```python
from build123d import *
from build123d.topology import SkipClean

# Parameters (mm, degrees)
CROQUIS2_R            = 2
CORTAR_EXTRUIR1_DEPTH = 5
REVOLUCI_N2_ANGLE     = 1.5
REVOLUCI_N3_ANGLE     = 1.5
MATRIZC1_COUNT        = 3


with BuildPart() as part:
    # Croquis1 → Revoluci_n1 (revolve)
    with BuildSketch(Plane.XY, mode=Mode.PRIVATE) as revoluci_n1_sk:
        Polygon((0, 56), (0, 90), (3.000002354, 90), (3.000002354, 60.169848481), (10.200002354, 60.169848481), (13.157056275, 57.212794561), (18.657056275, 57.212794561), (41.284473273, 34.585377563), (41.284473273, 32.888321288), (18.16, 56.012794561), (12.66, 56.012794561), (9.70294608, 58.969848481), (3.469848481, 58.969848481), (0.5, 56), align=None)
    revolve(revoluci_n1_sk.sketch.rotate(Axis((-46.033893017, 0, 0), (1, 0, 0)), 90), axis=Axis((-46.033893017, 0, 0), (1, 0, 0)))

    # Croquis2 → Cortar-Extruir1 (cut)
    with SkipClean():  # the faces are left unmerged after this step: merging them gives an invalid solid
        with BuildSketch(Plane.ZY):
            with Locations((63.219854476, 36.5)):
                Circle(CROQUIS2_R)
            with Locations((0, -73)):
                Circle(CROQUIS2_R)
            with Locations((-63.219854476, 36.5)):
                Circle(CROQUIS2_R)
            with BuildLine():
                Line((-14.422814665, 52.006989551), (-15.759006546, 56.825141817))
                ThreePointArc((-15.759006546, 56.825141817), (0, 58.969848481), (15.759006546, 56.825141817))
                Line((15.759006546, 56.825141817), (14.422814665, 52.006989551))
                ThreePointArc((14.422814665, 52.006989551), (0, 53.969848481), (-14.422814665, 52.006989551))
            make_face()
            with BuildLine():
                Line((52.250781458, -13.512970881), (57.09151966, -14.764870902))
                ThreePointArc((57.09151966, -14.764870902), (51.069386842, -29.48492424), (41.332513115, -42.060270916))
                Line((41.332513115, -42.060270916), (37.827966793, -38.49401867))
                ThreePointArc((37.827966793, -38.49401867), (46.739259823, -26.98492424), (52.250781458, -13.512970881))
            make_face()
            with BuildLine():
                Line((-37.827966793, -38.49401867), (-41.332513115, -42.060270916))
                ThreePointArc((-41.332513115, -42.060270916), (-51.069386842, -29.48492424), (-57.09151966, -14.764870902))
                Line((-57.09151966, -14.764870902), (-52.250781458, -13.512970881))
                ThreePointArc((-52.250781458, -13.512970881), (-46.739259823, -26.98492424), (-37.827966793, -38.49401867))
            make_face()
        extrude(amount=-CORTAR_EXTRUIR1_DEPTH, mode=Mode.SUBTRACT)

    # Croquis3 → Revoluci_n2 (revolve)
    with SkipClean():  # the faces are left unmerged after this step: merging them gives an invalid solid
        with BuildSketch(Plane(origin=(0, 0, 0), x_dir=(1, 0, 0), z_dir=(0, -0.9681476403781081, 0.2503800040544404))):
            Polygon((0.5, -56), (12.66, -56.012794561), (9.70294608, -58.969848481), (3.469848481, -58.969848481), align=None)
        revoluci_n2 = revolve(axis=Axis((9.70294608, 0, 0), (1, 0, 0)), revolution_arc=REVOLUCI_N2_ANGLE)

    # Croquis5 → Revoluci_n3 (revolve)
    with SkipClean():  # the faces are left unmerged after this step: merging them gives an invalid solid
        with BuildSketch(Plane(origin=(0, 0, 0), x_dir=(-1, 0, 0), z_dir=(0, -0.9504873560590977, -0.31076323137042167))):
            Polygon((-0.5, 56.012794561), (-3.469848481, 58.969848481), (-9.70294608, 58.969848481), (-12.66, 56.012794561), align=None)
        revoluci_n3 = revolve(axis=Axis((9.70294608, 0, 0), (1, 0, 0)), revolution_arc=REVOLUCI_N3_ANGLE)

    # MatrizC1: Revoluci_n2, Revoluci_n3 ×3 about axis
    with SkipClean():  # the faces are left unmerged after this step: merging them gives an invalid solid
        matrizc1_axis = Axis((0, 0, 0), (1, 0, 0))
        add([revoluci_n2.rotate(matrizc1_axis, i * 360 / MATRIZC1_COUNT) for i in range(1, MATRIZC1_COUNT)])
        add([revoluci_n3.rotate(matrizc1_axis, i * 360 / MATRIZC1_COUNT) for i in range(1, MATRIZC1_COUNT)])


solid = part.part
```
CAD build for the part. Positions are in the model's coordinates, mm. A direction names the side the tool comes from. Round coordinates to 2 decimals unless told otherwise and drop trailing zeros. Order: outer loops, then holes, each group sorted by start corner. A loop starts at its lowest first (then second) coordinate and runs counter-clockwise, first axis right, second up. Notation, with made-up numbers: (-10.75, -27) - (27.25, -27) arc R25 cw to (27.25, 10) - close; hole circle Ø10 at (-37.5, 67.5). An arc over 180 degrees is marked (long way). Answer in a Markdown table with one row per item. Add a question column.
(1) Mould opens along Y. For faces 1 (the face through (12.475, 49.597, -26.425)), 2 (the face through (0, -41, -39)), 3 (the face through (11.489, 48.316, 30.586)), 4 (the face through (15.946, 50.758, 26.4)) say: +Y half, -Y half, draft (parallel to the pull), parting line (faces both ways), or undercut.
(2) Drop flat-ended pins along their axis: pin 1 Ø1.5 at (y, z) = (42, -23) entering from +X; pin 2 Ø12 at (x, z) = (20, 10.5) entering from -Y; pin 3 Ø6 at (y, z) = (30, -4.5) entering from +X; pin 4 Ø5 at (y, z) = (36.5, -63.22) entering from +X. Give the stop position or say it passes through.
(3) Probe L1, parallel to X at y = 74, z = -47; L2, parallel to Y at x = 14, z = 0; L3, parallel to Z at x = 34.5, y = 0.5. List the from-to ranges inside material, lowest first. Write a range as [from, to].
(4) Band-saw the part on A-A on x = 37.5. List the corners of the cut face in (y, z), and give its area (3 significant figures).
(5) 3-axis set-ups, long thin cutter, end or side, ignore diameter. For faces 5 (the face through (0.246, -55.997, 0.609)), 6 (the face through (11.489, 2.33, -57.136)), 7 (the face through (1, -71, 0)), 8 (the face through (6.65, -18.073, 57.391)): which of +Z, -Z, +X, -X, +Y, -Y reach the whole face in a straight line?
(6) Band-saw the part on B-B on z = -69. List the corners of the cut face in (x, y).
(7) Band-saw the part on C-C on y = -62.5. List the corners of the cut face in (x, z).
Data:
| question | item | result |
|---|---|---|
| 1 | face 1 | undercut |
| 1 | face 2 | draft |
| 1 | face 3 | undercut |
| 1 | face 4 | parting line |
| 2 | pin 1 | stops at x = 28.73 |
| 2 | pin 2 | stops at y = -57.02 |
| 2 | pin 3 | stops at x = 41.28 |
| 2 | pin 4 | stops at x = 3 |
| 3 | L1 | x = [0, 3] |
| 3 | L2 | y = [-57.21, -56.01], [56.01, 57.21] |
| 3 | L3 | z = [-41.37, -39.67], [39.67, 41.37] |
| 4 | outline | circle Ø76.74 at (0, 0); hole circle Ø73.35 at (0, 0) |
| 4 | area | 400 mm^2 |
| 5 | face 5 | -X |
| 5 | face 6 | none |
| 5 | face 7 | +X, -X |
| 5 | face 8 | +X |
| 6 | outline | (0, -57.78) - (3, -57.78) - (3, 57.78) - (0, 57.78) - close |
| 7 | outline | (0, -64.76) - (3, -64.76) - (3, 64.76) - (0, 64.76) - close |
